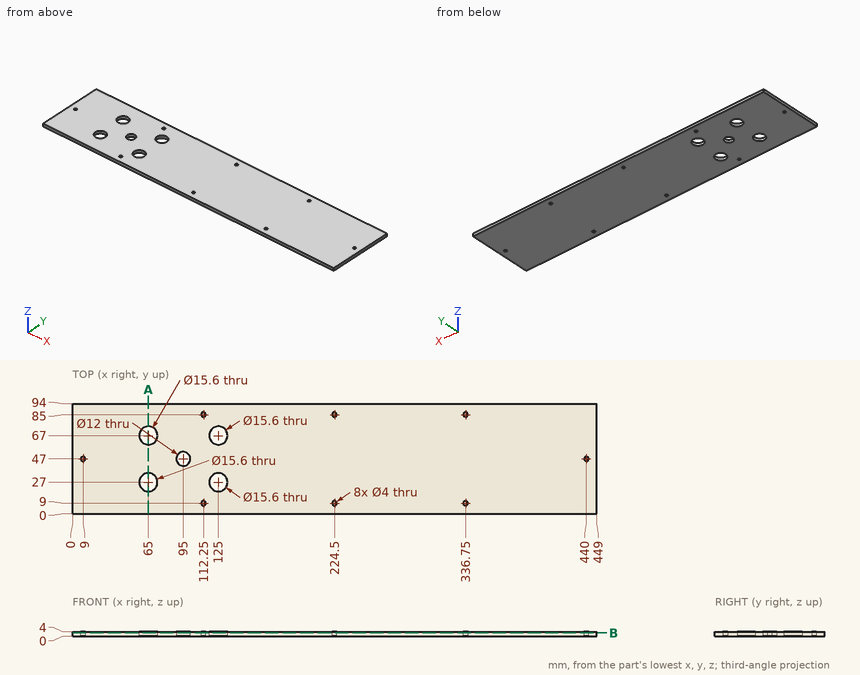
Drawing for the job (mm, zero at the part's lowest x, y, z). Round coordinates to 2 decimals unless told otherwise and drop trailing zeros. Loops run counter-clockwise (first coordinate to the right, second up) from the corner with the lowest first, then second, coordinate; pieces in that order, holes last.
1. Band-saw the part on B-B, the plane z = 2.95. Count the separate pieces of the cut face and the enclosed holes in it, and give its area (3 significant figures).
Check values:
separate pieces: 1
enclosed holes: 13
area: 41,200 mm2
2. Wall check: probe 1 along X at (y, z) = (46.5, 2.7); probe 2 along Y at (x, z) = (125, 1.9); probe 3 along X at (y, z) = (31, 1.7). Give the ranges that are in metal, low to high.
Check values:
probe 1: x = 0 to 7.06, 10.94 to 89.02, 100.98 to 438.06, 441.94 to 449
probe 2: y = 0 to 19.2, 34.8 to 59.2, 74.8 to 94
probe 3: x = 0 to 58.3, 71.7 to 118.3, 131.7 to 449
3. Band-saw the part on A-A, the plane x = 65. List the corners of the cut face in (y, z).
Check values:
outline: (0, 0) - (19.2, 0) - (19.2, 4) - (0, 4) - close; (34.8, 0) - (59.2, 0) - (59.2, 4) - (34.8, 4) - close; (74.8, 0) - (94, 0) - (94, 4) - (74.8, 4) - close
4. Drop a flat-ended pin along its axis: P1, Ø5, axis at x = 112.25, y = 85, coming from the +Z side. Give the stop position or say it passes through.
Check values:
P1: stops at z = 4
